```python
from build123d import *

# Parameters (mm, degrees)
F0_W     = 200
F0_H     = 90
F1_DEPTH = 8
F2_W     = 200
F2_H     = 15
F3_DEPTH = 30
F4_W     = 1.5
F4_H     = 126.118213
F4_H_2   = 132.641569
F5_DEPTH = 30.5


with BuildPart() as f1:
    # F0 (on Top) → F1 (new body)
    with BuildSketch(Plane.XY):
        Rectangle(F0_W, F0_H)
    extrude(amount=F1_DEPTH)

    # F2 (on face) → F3 (join)
    with BuildSketch(Plane.XY.offset(8)):
        with Locations((0, 37.5)):
            Rectangle(F2_W, F2_H)
        with Locations((0, -37.5)):
            Rectangle(F2_W, F2_H)
    extrude(amount=F3_DEPTH)

    # F4 (on face) → F5 (cut)
    with BuildSketch(Plane.XY.offset(38)):
        Polygon((0.75, 60), (-0.75, 60), (-0.75, 1.81066), (0, 1.06066), (0.75, 1.81066), align=None)
        Polygon((0, 1.06066), (-0.75, 1.81066), (-47.126677, 48.187338), (-48.187338, 47.126677), (-1.06066, 0), (-47.126677, -46.066017), (-46.066017, -47.126677), (-0.75, -1.81066), (0, -1.06066), (0.75, -1.81066), (57.87868, -58.93934), (58.93934, -57.87868), (1.06066, 0), (60, 58.93934), (58.93934, 60), (0.75, 1.81066), align=None)
        Polygon((0, -1.06066), (-0.75, -1.81066), (-0.75, -70), (0.75, -70), (0.75, -1.81066), align=None)
        with Locations((-74.25, -3.795997)):
            Rectangle(F4_W, F4_H)
        with Locations((74.25, -6.622784)):
            Rectangle(F4_W, F4_H_2)
    extrude(amount=-F5_DEPTH, mode=Mode.SUBTRACT)


solid = f1.part
```
Geometry: final body of the model. Coordinates: model frame, mm. A direction names the side the tool comes from. Coordinates: 2 decimals unless noted, no trailing zeros. Loops run counter-clockwise (first coordinate to the right, second up) from the corner with the lowest first, then second, coordinate; pieces in that order, holes last. Notation, with made-up numbers: (-10, 51.25) -> (33, 51.25) arc R29 ccw to (33, 72.25) -> close; hole circle Ø5 at (74.5, 2). An arc over 180 degrees is marked (long way). Use a Markdown table: item, result. Add a question column.
(1) Section query C-C, the plane z = 14.5. State how many separate pieces and enclosed holes the cut face has, plus the area to 3 significant figures.
(2) Line query: line 1 along Y through (x, z) = (53.5, 17); line 2 along Y through (x, z) = (43, 13.5); line 3 along X through (y, z) = (38, 35.5). Output: solid intervals per line, ascending.
(3) Section query B-B, the plane y = 34. Return loops of the section in (x, z).
(4) Pin query (flat end, axial travel): pin 1 Ø1.2 at (x, y) = (74, 15) entering from +Z. Return the tip coordinate at first contact, or that it passes through.
(5) Mould query, pull axis Y, two halves, no side actions, for faces 5 (the flat face through (-1, -45, 19)), 6 (the flat face through (-53, -30, 23)), 7 (the flat face through (57, 38, 38)). Classes: pulls with the +Y half, pulls with the -Y half, needs draft (parallel to the pull), parting line crosses it, or undercut.
(6) Section query D-D, the plane y = 12. Return loops of the section in (x, z).
(7) Access query for faces 1 (the flat face through (-0.75, -38, 24)), 2 (the flat face through (38.67, -37.61, 23.95)), 3 (the flat face through (17, 38, 38)), 4 (the flat face through (87, -30, 23)). Directions: +Z, -Z, +X, -X, +Y, -Y. A direction counts if a zero-diameter tool reaches every point of the face in a straight line with its end or side. Return the directions, or none.
(8) Section query A-A, the plane x = -70. Return loops of the section in (y, z), plus the area to 3 significant figures.
Answer:
| question | item | result |
|---|---|---|
| 1 | separate pieces | 12 |
| 1 | enclosed holes | 0 |
| 1 | area | 5,740 mm^2 |
| 2 | line 1 | y = -45 to -30, 30 to 45 |
| 2 | line 2 | y = -45 to -44.06, -41.94 to -30, 30 to 41.94, 44.06 to 45 |
| 2 | line 3 | x = -100 to -75, -73.5 to -39.06, -36.94 to -0.75, 0.75 to 36.94, 39.06 to 73.5, 75 to 100 |
| 3 | outline | (-100, 0) -> (100, 0) -> (100, 38) -> (75, 38) -> (75, 7.5) -> (73.5, 7.5) -> (73.5, 38) -> (35.06, 38) -> (35.06, 7.5) -> (32.94, 7.5) -> (32.94, 38) -> (0.75, 38) -> (0.75, 7.5) -> (-0.75, 7.5) -> (-0.75, 38) -> (-32.94, 38) -> (-32.94, 7.5) -> (-35.06, 7.5) -> (-35.06, 38) -> (-73.5, 38) -> (-73.5, 7.5) -> (-75, 7.5) -> (-75, 38) -> (-100, 38) -> close |
| 4 | pin 1 | stops at z = 8 |
| 5 | face 5 | pulls with the -Y half |
| 5 | face 6 | undercut |
| 5 | face 7 | needs draft |
| 6 | outline | (-100, 0) -> (100, 0) -> (100, 8) -> (75, 8) -> (75, 7.5) -> (73.5, 7.5) -> (73.5, 8) -> (13.06, 8) -> (13.06, 7.5) -> (10.94, 7.5) -> (10.94, 8) -> (0.75, 8) -> (0.75, 7.5) -> (-0.75, 7.5) -> (-0.75, 8) -> (-10.94, 8) -> (-10.94, 7.5) -> (-13.06, 7.5) -> (-13.06, 8) -> (-73.5, 8) -> (-73.5, 7.5) -> (-75, 7.5) -> (-75, 8) -> (-100, 8) -> close |
| 7 | face 1 | +Z, +Y, -Y |
| 7 | face 2 | +Z |
| 7 | face 3 | +Z, +X, -X, +Y, -Y |
| 7 | face 4 | +Z, +X, -X |
| 8 | outline | (-45, 0) -> (45, 0) -> (45, 38) -> (30, 38) -> (30, 8) -> (-30, 8) -> (-30, 38) -> (-45, 38) -> close |
| 8 | area | 1,620 mm^2 |
